Design review of the part built by this model. Coordinates are the model's own, in mm. Face numbers are marked on the shaded views. A direction names the side the tool comes from. Give positions to 0.01 mm unless a question says otherwise; leave off trailing zeros. Order: outer loops, then holes, each group sorted by start corner. A loop starts at its lowest first (then second) coordinate and runs counter-clockwise, first axis right, second up.
```python
from build123d import *

# Parameters (mm, degrees)
SKETCH_1_W          = 3
SKETCH_1_H          = 17
SKETCH_1_H_2        = 3
SKETCH_1_W_2        = 27
EXTRUDE_1_DEPTH     = 50
SKETCH_2_R          = 2
CUT_EXTRUDE_1_DEPTH = 10
CUT_EXTRUDE_2_DEPTH = 10


with BuildPart() as part:
    # 草图1 → 凸台-拉伸1 (new body)
    with BuildSketch(Plane(origin=(0, 0, 0), x_dir=(1, 0, 0), z_dir=(0, 1, 0))):
        with Locations((0, 1.5)):
            Rectangle(SKETCH_1_W, SKETCH_1_H)
        with Locations((0, -8.5)):
            Rectangle(SKETCH_1_W, SKETCH_1_H_2)
        with Locations((15, -8.5)):
            Rectangle(SKETCH_1_W_2, SKETCH_1_H_2)
    extrude(amount=EXTRUDE_1_DEPTH)

    # 草图2 → 切除-拉伸1 (cut)
    with BuildSketch(Plane.XY.offset(10)):
        with Locations((21.5, 36.8)):
            Circle(SKETCH_2_R)
        with Locations((21.5, 24.1)):
            Circle(SKETCH_2_R)
        with Locations((21.5, 11.4)):
            Circle(SKETCH_2_R)
    extrude(amount=-CUT_EXTRUDE_1_DEPTH, mode=Mode.SUBTRACT)

    # 草图3 → 切除-拉伸2 (cut)
    with BuildSketch(Plane.ZY.offset(1.5)):
        with BuildLine():
            Line((1, 40), (1, 10))
            ThreePointArc((1, 10), (-3, 6), (-7, 10))
            Line((-7, 10), (-7, 40))
            ThreePointArc((-7, 40), (-3, 44), (1, 40))
        make_face()
    extrude(amount=-CUT_EXTRUDE_2_DEPTH, mode=Mode.SUBTRACT)


solid = part.part
```
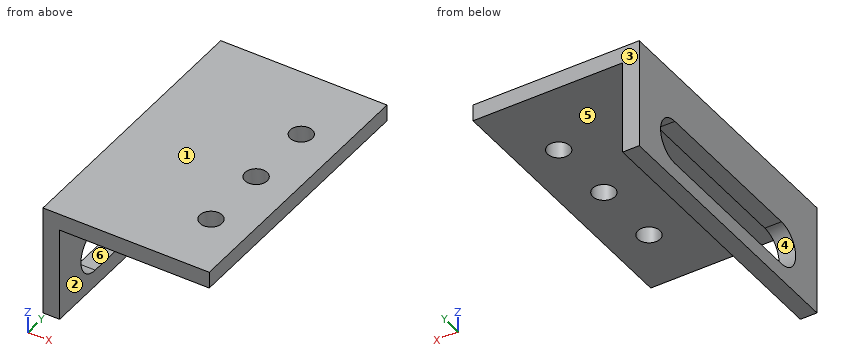
1. Draft analysis for pull direction Y (two halves, no side actions). For the marked faces 3, 4, 5 and 6, state which applies: pulls with the +Y half, pulls with the -Y half, needs draft (parallel to the pull), parting line crosses it, or undercut.
Recorded:
face 3: pulls with the +Y half
face 4: undercut
face 5: needs draft
face 6: undercut
2. For pin 1 (8.5 mm diameter, centred on y = 18.5, z = -2.5, fed in from +X); pin 2 (13.5 mm diameter, centred on x = 20.5, y = 34, fed in from -Z); pin 3 (4 mm diameter, centred on y = 20, z = 0.5, fed in from -X); pin 4 (6 mm diameter, centred on x = 19.5, z = 3, fed in from -Y), all flat-tipped, find the tip position at first contact; note any pin that passes through.
Recorded:
pin 1: stops at x = 1.5
pin 2: stops at z = 7
pin 3: stops at x = -1.5
pin 4: passes through
3. Take a section at D-D (y = 29). State the section outline as (x, z) points.
Recorded:
outline: (-1.5, -10) - (1.5, -10) - (1.5, -7) - (-1.5, -7) - close; (-1.5, 1) - (1.5, 1) - (1.5, 7) - (28.5, 7) - (28.5, 10) - (-1.5, 10) - close
4. Take a section at C-C (x = 21.5). State the section outline as (y, z) points.
Recorded:
outline: (0, 7) - (9.4, 7) - (9.4, 10) - (0, 10) - close; (13.4, 7) - (22.1, 7) - (22.1, 10) - (13.4, 10) - close; (26.1, 7) - (34.8, 7) - (34.8, 10) - (26.1, 10) - close; (38.8, 7) - (50, 7) - (50, 10) - (38.8, 10) - close
5. For line 1 along Y through (x, z) = (21.5, 7.7); line 2 along Z through (x, y) = (1.25, 20.5); line 3 along Z through (x, y) = (6.25, 2), list the stretches that pass through material, from the lowest coordinate up.
Recorded:
line 1: y = 0 to 9.4, 13.4 to 22.1, 26.1 to 34.8, 38.8 to 50
line 2: z = -10 to -7, 1 to 10
line 3: z = 7 to 10
6. Take a section at B-B (z = 8). State the section outline as (x, y) points.
Recorded:
outline: (-1.5, 0) - (28.5, 0) - (28.5, 50) - (-1.5, 50) - close; hole circle Ø4 at (21.5, 11.4); hole circle Ø4 at (21.5, 24.1); hole circle Ø4 at (21.5, 36.8)
7. Machinability: for the marked faces 1 and 2, which of the approach directions +Z, -Z, +X, -X, +Y, -Y give a long, thin tool a straight path to every point of the face, cutting with its end or side? Answer none if there is none.
Recorded:
face 1: +Z, +X, -X, +Y, -Y
face 2: -Z, +X, +Y, -Y
8. Take a section at A-A (y = 36.8). State the section outline as (x, z) points, then the cut area to 3 significant figures.
Recorded:
outline: (-1.5, -10) - (1.5, -10) - (1.5, -7) - (-1.5, -7) - close; (-1.5, 1) - (1.5, 1) - (1.5, 7) - (19.5, 7) - (19.5, 10) - (-1.5, 10) - close; (23.5, 7) - (28.5, 7) - (28.5, 10) - (23.5, 10) - close
area: 105 mm2
